from build123d import *

# Parameters (mm, degrees)
SKETCH2_W           = 20.1
SKETCH2_H           = 3.25
BOSS_EXTRUDE1_DEPTH = 3.15
FILLET1_R           = 50
SKETCH5_W           = 20
SKETCH5_H           = 3.16
CUT_EXTRUDE2_DEPTH  = 255.013877696
SKETCH7_R           = 1.4
CUT_EXTRUDE3_DEPTH  = 255.013877696
SKETCH8_R           = 1.4
CUT_EXTRUDE4_DEPTH  = 10
SKETCH10_R          = 1.4
CUT_EXTRUDE5_DEPTH  = 10
SKETCH11_W          = 3.79
SKETCH11_H          = 3.19
CUT_EXTRUDE6_DEPTH  = 10


with BuildPart() as part:
    # Sketch2 → Boss-Extrude1 (new body)
    with BuildSketch(Plane(origin=(0, 0, 0), x_dir=(1, 0, 0), z_dir=(0, 1, 0))):
        Polygon((-199.52829939, 76.482620099), (-157.52829939, 76.482620099), (-157.52829939, -113.167379901), (-199.52829939, -113.167379901), (-199.52829939, -157.167379901), (60.67170061, -157.167379901), (60.67170061, 120.482620099), (-199.52829939, 120.482620099), align=None)
        with Locations((-95.774503115, 105.482620099)):
            Rectangle(SKETCH2_W, SKETCH2_H, mode=Mode.SUBTRACT)
        with Locations((-135.774503115, -142.167379901)):
            Rectangle(SKETCH2_W, SKETCH2_H, mode=Mode.SUBTRACT)
        with Locations((-95.774503115, -142.167379901)):
            Rectangle(SKETCH2_W, SKETCH2_H, mode=Mode.SUBTRACT)
        with Locations((-135.774503115, 105.482620099)):
            Rectangle(SKETCH2_W, SKETCH2_H, mode=Mode.SUBTRACT)
    extrude(amount=BOSS_EXTRUDE1_DEPTH)

    # Fillet1
    # the kernel refuses this fillet: 50 mm, written as the material it takes off along each edge
    with BuildSketch(Plane(origin=(-199.52829939, -124.09673646, -120.482620099), x_dir=(1, 0, 0), z_dir=(0, 1, 0))) as fillet1_piece_1:
        with BuildLine():
            CenterArc((49.638694584, -50), FILLET1_R, 90, 83.107897421)
            Line((0, -44), (-0.992773892, -43.88))
            ThreePointArc((-0.992773892, -43.88), (-1, -22), (-1, 0))
            Line((-1, 0), (0, 1))
            Line((0, 1), (49.638694584, 1))
            Line((49.638694584, 1), (49.638694584, 0))
        make_face()
    extrude(amount=251.34347292, mode=Mode.SUBTRACT)
    with BuildSketch(Plane(origin=(-199.52829939, -124.09673646, 157.167379901), x_dir=(0, 0, -1), z_dir=(0, 1, 0))) as fillet1_piece_2:
        with BuildLine():
            CenterArc((50, -49.638694584), FILLET1_R, 96.892102579, 83.107897421)
            Line((0, -49.638694584), (-1, -49.638694584))
            Line((-1, -49.638694584), (-1, 0))
            Line((-1, 0), (0, 1))
            ThreePointArc((0, 1), (22, 1), (43.88, 0.992773892))
            Line((43.88, 0.992773892), (44, 0))
        make_face()
    extrude(amount=251.34347292, mode=Mode.SUBTRACT)

    # Sketch5 → Cut-Extrude2 (cut, through all)
    with BuildSketch(Plane(origin=(0, 0, 0), x_dir=(1, 0, 0), z_dir=(0, 1, 0))):
        with Locations((-94.42829939, 118.902620099)):
            Rectangle(SKETCH5_W, SKETCH5_H)
        with Locations((-134.42829939, 118.902620099)):
            Rectangle(SKETCH5_W, SKETCH5_H)
        with Locations((-54.42829939, 118.902620099)):
            Rectangle(SKETCH5_W, SKETCH5_H)
        with Locations((-14.42829939, 118.902620099)):
            Rectangle(SKETCH5_W, SKETCH5_H)
        with Locations((25.57170061, 118.902620099)):
            Rectangle(SKETCH5_W, SKETCH5_H)
        with Locations((25.57170061, -155.587379901)):
            Rectangle(SKETCH5_W, SKETCH5_H)
        with Locations((-14.42829939, -155.587379901)):
            Rectangle(SKETCH5_W, SKETCH5_H)
        with Locations((-54.42829939, -155.587379901)):
            Rectangle(SKETCH5_W, SKETCH5_H)
        with Locations((-94.42829939, -155.587379901)):
            Rectangle(SKETCH5_W, SKETCH5_H)
        with Locations((-134.42829939, -155.587379901)):
            Rectangle(SKETCH5_W, SKETCH5_H)
    extrude(amount=CUT_EXTRUDE2_DEPTH, mode=Mode.SUBTRACT)

    # Sketch7 → Cut-Extrude3 (cut, through all)
    with BuildSketch(Plane.XZ):
        with Locations(Location((23.12170061, 148.342379901, 0), (0, 0, 270))):
            Circle(SKETCH7_R)
        with Locations(Location((53.12170061, 148.342379901, 0), (0, 0, 270))):
            Circle(SKETCH7_R)
        with Locations(Location((53.12170061, -111.657620099, 0), (0, 0, 90))):
            Circle(SKETCH7_R)
        with Locations(Location((23.12170061, -111.657620099, 0), (0, 0, 90))):
            Circle(SKETCH7_R)
    extrude(amount=-CUT_EXTRUDE3_DEPTH, mode=Mode.SUBTRACT)

    # Sketch8 → Cut-Extrude4 (cut)
    with BuildSketch(Plane.XZ):
        with Locations(Location((-177.812570637, 135.451651148, 0), (0, 0, 270))):
            Circle(SKETCH8_R)
        with Locations(Location((-177.812570637, -98.766891346, 0), (0, 0, 270))):
            Circle(SKETCH8_R)
    extrude(amount=-CUT_EXTRUDE4_DEPTH, mode=Mode.SUBTRACT)

    # Sketch10 → Cut-Extrude5 (cut)
    with BuildSketch(Plane(origin=(0, 3.15, 0), x_dir=(1, 0, 0), z_dir=(0, 1, 0))):
        with Locations(Location((-144.129756514, -123.342379901, 0), (0, 0, 270))):
            Circle(SKETCH10_R)
        with Locations(Location((-144.129756514, 86.657620099, 0), (0, 0, 270))):
            Circle(SKETCH10_R)
        with Locations(Location((-144.129756514, 51.657620099, 0), (0, 0, 270))):
            Circle(SKETCH10_R)
        with Locations(Location((-144.129756514, 16.657620099, 0), (0, 0, 270))):
            Circle(SKETCH10_R)
        with Locations(Location((-144.129756514, -18.342379901, 0), (0, 0, 270))):
            Circle(SKETCH10_R)
        with Locations(Location((-144.129756514, -53.342379901, 0), (0, 0, 270))):
            Circle(SKETCH10_R)
        with Locations(Location((-144.129756514, -88.342379901, 0), (0, 0, 270))):
            Circle(SKETCH10_R)
    extrude(amount=-CUT_EXTRUDE5_DEPTH, mode=Mode.SUBTRACT)

    # Sketch11 → Cut-Extrude6 (cut)
    with BuildSketch(Plane.XZ):
        with Locations((-87.319899774, -102.332620099)):
            Rectangle(SKETCH11_W, SKETCH11_H)
        with Locations((-81.069899774, -102.332620099)):
            Rectangle(SKETCH11_W, SKETCH11_H)
        with Locations((-87.319899774, 139.017379901)):
            Rectangle(SKETCH11_W, SKETCH11_H)
        with Locations((-81.069899774, 139.017379901)):
            Rectangle(SKETCH11_W, SKETCH11_H)
    extrude(amount=-CUT_EXTRUDE6_DEPTH, mode=Mode.SUBTRACT)


solid = part.part
Source: CAD feature listing. Evaluate the final solid. Frame: model axes, mm. Round coordinates to 2 decimals unless told otherwise and drop trailing zeros. Order: outer loops, then holes, each group sorted by start corner. A loop starts at its lowest first (then second) coordinate and runs counter-clockwise, first axis right, second up. Notation, with made-up numbers: (79.25, -6.75) - (99.25, -6.75) arc R14 ccw to (99.25, 17.25) - close; hole circle Ø2 at (73.25, 6). An arc over 180 degrees is marked (long way). Use a Markdown table: item, result. Add a question column.
1. Section query D-D (x = -20.5). Return the cut outline in (y, z), then the cut area to 3 significant figures.
2. Section query B-B (z = 27). Return the cut outline in (x, y).
3. Section query C-C (y = 2.6). Give the number of separate pieces and of enclosed holes in the cut face, then the cut area to 3 significant figures.
4. Section query A-A (x = -168.5). Return the cut outline in (y, z).
5. Line query: probe 1 along Z at (x, y) = (-130, 2.9); probe 2 along X at (y, z) = (1, -101); probe 3 along X at (y, z) = (0.45, -106.5). Output: solid intervals per line, ascending.
6. First-contact query: pin 1 (0.9 mm diameter, centred on x = -88, y = 2, fed in from +Z); pin 2 (0.9 mm diameter, centred on y = 2.5, z = -102.5, fed in from -X); pin 3 (1 mm diameter, centred on y = 2.5, z = -42, fed in from -X). Flat tips, straight axial feed; report the tip coordinate or a pass-through.
Derived:
| question | item | result |
|---|---|---|
| 1 | outline | (0, -117.32) - (3.15, -117.32) - (3.15, 154.01) - (0, 154.01) - close |
| 1 | area | 855 mm2 |
| 2 | outline | (-157.53, 0) - (60.67, 0) - (60.67, 3.15) - (-157.53, 3.15) - close |
| 3 | separate pieces | 1 |
| 3 | enclosed holes | 19 |
| 3 | area | 62,200 mm2 |
| 4 | outline | (0, -116.89) - (3.15, -116.89) - (3.15, -76.48) - (0, -76.48) - close; (0, 113.17) - (3.15, 113.17) - (3.15, 153.57) - (0, 153.57) - close |
| 5 | probe 1 | -117.32 to -107.11, -103.86 to 140.54, 143.79 to 154.01 |
| 5 | probe 2 | -189.5 to -89.21, -85.42 to -82.96, -79.17 to 60.67 |
| 5 | probe 3 | -184.57 to -145.82, -125.72 to -105.82, -85.72 to 60.67 |
| 6 | pin 1 | z = 154.01 |
| 6 | pin 2 | x = -188.66 |
| 6 | pin 3 | x = -157.53 |
